For this review, take the finished solid that the model builds, in its own axes (mm). A direction names the side the tool comes from. Coordinates: 2 decimals unless noted, no trailing zeros. Write each loop counter-clockwise with the first axis right and the second up, starting at its lowest first coordinate (ties: lowest second). Pieces come first, ordered by that corner, then holes. Notation, with made-up numbers: (-33, -17) - (23, -17) arc R17 cw to (23, 11) - close; hole circle Ø11 at (73.5, -5). An arc over 180 degrees is marked (long way). Write each question's results on one line, items separated by ' | '.
from build123d import *
from build123d.topology import SkipClean

# Parameters (mm, degrees)
SKETCH_1_R          = 1.5
SKETCH_1_R_2        = 6
SKETCH_1_R_3        = 1.2
EXTRUDE_3_DEPTH     = 5
SKETCH_1_128_R      = 2.1
SKETCH_1_128_R_2    = 2.694546499
CUT_EXTRUDE_1_DEPTH = 3


with BuildPart() as part:
    # Sketch 1 → Extrude 3 (new body)
    with BuildSketch(Plane.XY):
        with BuildLine():
            ThreePointArc((-50, -28.867513459), (0, -42.264973081), (50, -28.867513459))
            ThreePointArc((50, -28.867513459), (36.602540378, 21.132486541), (0, 57.735026919))
            ThreePointArc((0, 57.735026919), (-36.602540378, 21.132486541), (-50, -28.867513459))
        make_face()
        with Locations((-46, -26.558112383)):
            Circle(SKETCH_1_R, mode=Mode.SUBTRACT)
        with BuildLine():
            Line((-12.318904501, -4.627679794), (-7.681095499, -4.627679794))
            ThreePointArc((-7.681095499, -4.627679794), (-7.305700474, -6.036481484), (-7.719101931, -7.434602674))
            Line((-7.719101931, -7.434602674), (-12.280898069, -7.434602674))
            ThreePointArc((-12.280898069, -7.434602674), (-12.694299526, -6.036481484), (-12.318904501, -4.627679794))
        make_face(mode=Mode.SUBTRACT)
        Circle(SKETCH_1_R_2, mode=Mode.SUBTRACT)
        with BuildLine():
            ThreePointArc((-10.923034521, -11.691335119), (0.030725767, -15.999970498), (10.967857029, -11.649296639))
            Line((10.967857029, -11.649296639), (39.141662126, -24.608662006))
            ThreePointArc((39.141662126, -24.608662006), (40.887936946, -27.352330968), (39.108544771, -30.074638556))
            ThreePointArc((39.108544771, -30.074638556), (0.120715527, -38.389897283), (-38.887875634, -30.17258796))
            ThreePointArc((-38.887875634, -30.17258796), (-40.674081889, -27.456751691), (-38.938338523, -24.708389561))
            Line((-38.938338523, -24.708389561), (-10.923034521, -11.691335119))
        make_face(mode=Mode.SUBTRACT)
        with Locations((46, -26.558112383)):
            Circle(SKETCH_1_R, mode=Mode.SUBTRACT)
        with BuildLine():
            ThreePointArc((7.719101931, -7.434602674), (7.305700474, -6.036481484), (7.681095499, -4.627679794))
            Line((7.681095499, -4.627679794), (12.318904501, -4.627679794))
            ThreePointArc((12.318904501, -4.627679794), (12.694299526, -6.036481484), (12.280898069, -7.434602674))
            Line((12.280898069, -7.434602674), (7.719101931, -7.434602674))
        make_face(mode=Mode.SUBTRACT)
        with BuildLine():
            ThreePointArc((-4.584422556, 15.329157506), (-13.835670885, 8.03580806), (-15.586551128, -3.613782498))
            Line((-15.586551128, -3.613782498), (-40.867216831, -21.36673515))
            ThreePointArc((-40.867216831, -21.36673515), (-44.11523634, -21.495718376), (-45.57409004, -18.590892513))
            ThreePointArc((-45.57409004, -18.590892513), (-33.183543116, 19.304197945), (-6.482898448, 48.912289883))
            ThreePointArc((-6.482898448, 48.912289883), (-3.236245956, 49.092161401), (-1.732813457, 46.208969266))
            Line((-1.732813457, 46.208969266), (-4.57661325, 15.413723751))
            Line((-4.57661325, 15.413723751), (-4.584422556, 15.329157506))
        make_face(mode=Mode.SUBTRACT)
        with Locations((-6.616406845, 9.232315636)):
            Circle(SKETCH_1_R_3, mode=Mode.SUBTRACT)
        with Locations((0, 53.230084709)):
            Circle(SKETCH_1_R, mode=Mode.SUBTRACT)
        with BuildLine():
            ThreePointArc((15.57251534, -3.673794493), (13.855876537, 8.000917785), (4.60262837, 15.323700992))
            Line((4.60262837, 15.323700992), (4.594769235, 15.408321271))
            Line((4.594769235, 15.408321271), (1.734391802, 46.206359162))
            ThreePointArc((1.734391802, 46.206359162), (3.23701886, 49.090744976), (6.484377608, 48.91121571))
            ThreePointArc((6.484377608, 48.91121571), (33.24460594, 19.198599415), (45.599673385, -18.831673998))
            ThreePointArc((45.599673385, -18.831673998), (44.131781944, -21.73382662), (40.882557513, -21.593342745))
            Line((40.882557513, -21.593342745), (15.64187559, -3.722901655))
            Line((15.64187559, -3.722901655), (15.57251534, -3.673794493))
        make_face(mode=Mode.SUBTRACT)
        with Locations((6.616406845, 9.232315636)):
            Circle(SKETCH_1_R_3, mode=Mode.SUBTRACT)
    extrude(amount=EXTRUDE_3_DEPTH)

    # Sketch 1_128 → Cut-Extrude 1 (cut)
    with SkipClean():  # the faces are left unmerged after this step: merging them gives an invalid solid
        with BuildSketch(Plane.XY):
            with Locations((-6.616406845, 9.232315636)):
                Circle(SKETCH_1_128_R)
            with Locations((6.616406845, 9.232315636)):
                Circle(SKETCH_1_128_R)
            with Locations(Location((-10, -6, 0), (0, 0, 149.383090202))):
                Circle(SKETCH_1_128_R_2)
            with Locations(Location((10, -6, 0), (0, 0, 149.383090202))):
                Circle(SKETCH_1_128_R_2)
        extrude(amount=CUT_EXTRUDE_1_DEPTH, mode=Mode.SUBTRACT)


solid = part.part
Q1. For pin 1 (15.5 mm diameter, centred on x = 0, y = 0, fed in from +Z); pin 2 (1 mm diameter, centred on x = -9.5, z = 4, fed in from -Y); pin 3 (1 mm diameter, centred on x = -10.5, y = -8, fed in from -Z); pin 4 (2 mm diameter, centred on y = 1.5, z = 2.5, fed in from -X), all flat-tipped, find the tip position at first contact; note any pin that passes through.
Results found:
pin 1: z = 5 | pin 2: y = -41.86 | pin 3: z = 3 | pin 4: x = -45.59
Q2. For faces 4 (the face through (-36.23, 21.77, 2.46)), 5 (the face through (-7.07, 7.18, 1.48)), 6 (the face through (0, -16, 2)), list the 3-axis set-ups (+Z, -Z, +X, -X, +Y, -Y) from which the entire face can be reached by the end or side of a thin tool; tool diameter is ignored.
Results found:
face 4: +Z, -Z, -X, +Y | face 5: -Z | face 6: +Z, -Z
Q3. Take a section at C-C on y = -34. State the section outline as (x, z) points, plus the area to 3 significant figures.
Results found:
outline: (-39.81, 0) - (-28.72, 0) - (-28.72, 5) - (-39.81, 5) - close; (28.72, 0) - (39.81, 0) - (39.81, 5) - (28.72, 5) - close | area: 111 mm2
Q4. Take a section at D-D on y = 0. State the section outline as (x, z) points.
Results found:
outline: (-45.74, 0) - (-41.69, 0) - (-41.69, 5) - (-45.74, 5) - close; (-16, 0) - (-6, 0) - (-6, 5) - (-16, 5) - close; (6, 0) - (16, 0) - (16, 5) - (6, 5) - close; (41.69, 0) - (45.74, 0) - (45.74, 5) - (41.69, 5) - close
Q5. Wall thickness on line 1 along Y through (x, z) = (0, 4); line 2 along X through (y, z) = (-21.5, 1.05); line 3 along X through (y, z) = (-1.5, 3.95): over which ranges is each line inside the solid? List them lowest first. Write a range as from..to.
Results found:
line 1: -42.26..-38.39, -16..-6, 6..51.73, 54.73..57.74 | line 2: -49.73..-44.11, -41.07..-32.03, 32.38..40.75, 44.47..49.73 | line 3: -46.18..-42.15, -15.93..-5.81, 5.81..15.93, 42.15..46.18
Q6. Mouldability with a two-part tool opening along Y and no side actions: class faces 1 (the face through (8, 8, 3)), 2 (the face through (-4, -7, 5)), 3 (the face through (36.967, 20.496, 2.465)) as pulls with the +Y half, pulls with the -Y half, needs draft (parallel to the pull), parting line crosses it, or undercut.
Results found:
face 1: undercut | face 2: needs draft | face 3: pulls with the +Y half
Q7. Take a section at B-B on x = 34. State the section outline as (y, z) points, plus the area to 3 significant figures.
Results found:
outline: (-36.31, 0) - (-32.18, 0) - (-32.18, 5) - (-36.31, 5) - close; (-22.24, 0) - (-16.72, 0) - (-16.72, 5) - (-22.24, 5) - close; (17.87, 0) - (25.39, 0) - (25.39, 5) - (17.87, 5) - close | area: 85.9 mm2
Q8. Take a section at A-A on y = 24. State the section outline as (x, z) points, plus the area to 3 significant figures.
Results found:
outline: (-34.88, 0) - (-30.28, 0) - (-30.28, 5) - (-34.88, 5) - close; (-3.78, 0) - (3.8, 0) - (3.8, 5) - (-3.78, 5) - close; (30.28, 0) - (34.88, 0) - (34.88, 5) - (30.28, 5) - close | area: 83.9 mm2
